Source: CAD feature listing. Evaluate the final solid. Frame: model axes, mm. Face numbers are marked on the shaded views. A direction names the side the tool comes from. Coordinates: 2 decimals unless noted, no trailing zeros. Loops run counter-clockwise (first coordinate to the right, second up) from the corner with the lowest first, then second, coordinate; pieces in that order, holes last. Notation, with made-up numbers: (50.5, 34.5) -> (94.5, 34.5) arc R22 cw to (94.5, 40.5) -> close; hole circle Ø3 at (-32.5, 82). An arc over 180 degrees is marked (long way). Answer as a JSON object with one key per item and string values. Group by question number.
from build123d import *

# Parameters (mm, degrees)
SKETCH_W        = 150
SKETCH_H        = 100
PAD_DEPTH       = 60
POCKET_DEPTH    = 58
SKETCH002_R     = 3
PAD001_DEPTH    = 37.8
POCKET001_DEPTH = 2
POCKET002_DEPTH = 2
SKETCH007_R     = 1
POCKET003_DEPTH = 2.001
SKETCH009_R     = 1.5
PAD003_DEPTH    = 10
POCKET004_DEPTH = 6
POCKET005_DEPTH = 6
CHAMFER_ANGLE   = 60
CHAMFER_SIZE    = 4
FILLET_R        = 2
FILLET001_R     = 2


with BuildPart() as part:
    # Sketch → Pad (new body)
    with BuildSketch(Plane.XZ):
        with Locations((75, 50)):
            Rectangle(SKETCH_W, SKETCH_H)
    extrude(amount=PAD_DEPTH)

    # Sketch001 (on Face6 of Pad) → Pocket (cut)
    with BuildSketch(Plane.XZ.offset(60)):
        Polygon((2, 98), (148, 98), (148, 56), (142, 56), (142, 44), (148, 44), (148, 2), (2, 2), (2, 44), (8, 44), (8, 56), (2, 56), align=None)
    extrude(amount=-POCKET_DEPTH, mode=Mode.SUBTRACT)

    # Sketch002 (on Face19 of Pocket) → Pad001 (join)
    with BuildSketch(Plane.XZ.offset(2)):
        with Locations((24.75, 80)):
            Circle(SKETCH002_R)
        with Locations((95.75, 80)):
            Circle(SKETCH002_R)
        with Locations((24.75, 20)):
            Circle(SKETCH002_R)
        with Locations((95.75, 20)):
            Circle(SKETCH002_R)
    extrude(amount=PAD001_DEPTH)

    # Sketch005 → Pocket001 (cut)
    with BuildSketch(Plane(origin=(0, 0, 0), x_dir=(1, 0, 0), z_dir=(0, 0, -1))):
        with BuildLine():
            ThreePointArc((65, 13), (61, 9), (65, 5))
            Line((65, 5), (85, 5))
            ThreePointArc((85, 5), (89, 9), (85, 13))
            Line((65, 13), (85, 13))
        make_face()
    extrude(amount=-POCKET001_DEPTH, mode=Mode.SUBTRACT)

    # Sketch006 (on Face5 of Pocket001) → Pocket002 (cut)
    with BuildSketch(Plane(origin=(150, 0, 0), x_dir=(0, 0, 1), z_dir=(1, 0, 0))):
        with BuildLine():
            ThreePointArc((25, 35), (17.5, 42.5), (10, 35))
            Line((10, 35), (10, 25))
            ThreePointArc((10, 25), (17.5, 17.5), (25, 25))
            Line((25, 35), (25, 25))
        make_face()
    extrude(amount=-POCKET002_DEPTH, mode=Mode.SUBTRACT)

    # Sketch007 (on Face27 of Pocket002) → Pocket003 (cut, through all)
    with BuildSketch(Plane.XZ.offset(2)):
        with Locations((40, 50)):
            Circle(SKETCH007_R)
        with Locations((110, 50)):
            Circle(SKETCH007_R)
    extrude(amount=-POCKET003_DEPTH, mode=Mode.SUBTRACT)

    # Sketch009 (on Face35 of Pocket003) → Pad003 (join)
    with BuildSketch(Plane.XZ.offset(39.8)):
        with Locations((24.75, 80)):
            Circle(SKETCH009_R)
        with Locations((95.75, 80)):
            Circle(SKETCH009_R)
        with Locations((24.75, 20)):
            Circle(SKETCH009_R)
        with Locations((95.75, 20)):
            Circle(SKETCH009_R)
    extrude(amount=PAD003_DEPTH)

    # Sketch010 (on Face14 of Pad003) → Pocket004 (cut)
    with BuildSketch(Plane(origin=(0, 0, 56), x_dir=(-1, 0, 0), z_dir=(0, 0, 1))):
        Polygon((-3.75, 60), (-3.75, 57.3), (-2.75, 57.3), (-2.75, 51.7), (-7.25, 51.7), (-7.25, 57.3), (-6.25, 57.3), (-6.25, 60), align=None)
    extrude(amount=-POCKET004_DEPTH, mode=Mode.SUBTRACT)

    # Sketch011 (on Face24 of Pocket004) → Pocket005 (cut)
    with BuildSketch(Plane(origin=(0, 0, 56), x_dir=(-1, 0, 0), z_dir=(0, 0, 1))):
        Polygon((-143.75, 60), (-146.25, 60), (-146.25, 57.3), (-147.25, 57.3), (-147.25, 51.7), (-142.74998, 51.7), (-142.75, 57.3), (-143.75, 57.3), align=None)
    extrude(amount=-POCKET005_DEPTH, mode=Mode.SUBTRACT)

    # Chamfer
    chamfer_edges = [part.edges().sort_by_distance(p)[0] for p in [
        (21.75, -2, 80),
        (92.75, -2, 80),
        (92.75, -2, 20),
        (21.75, -2, 20),
    ]]
    chamfer_side = part.faces().sort_by_distance((75.121299, -2, 50))[0]
    chamfer(chamfer_edges, length=CHAMFER_SIZE, angle=CHAMFER_ANGLE, reference=chamfer_side)

    # Fillet
    fillet_edges = [part.edges().sort_by_distance(p)[0] for p in [
        (2, -31, 98),
        (2, -31, 2),
        (148, -31, 2),
        (148, -31, 98),
    ]]
    fillet(fillet_edges, radius=FILLET_R)

    # Fillet001
    fillet001_edges = [part.edges().sort_by_distance(p)[0] for p in [
        (0, -30, 0),
        (0, -30, 100),
        (150, -30, 100),
        (150, -30, 0),
    ]]
    fillet(fillet001_edges, radius=FILLET001_R)


solid = part.part
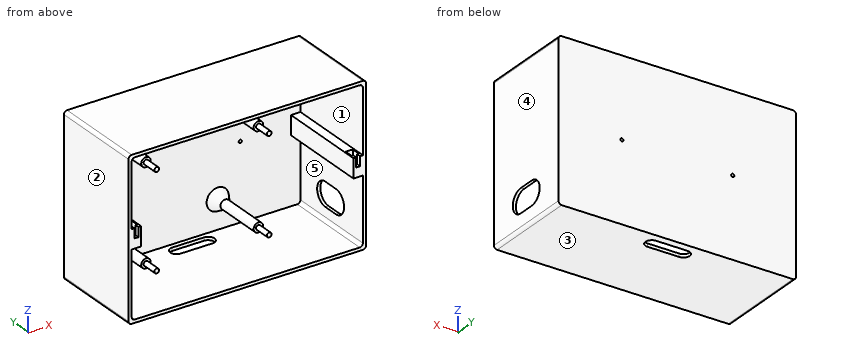
1. Reachability of the marked faces 1 and 2 from +Z, -Z, +X, -X, +Y, -Y: full face, straight path, thin tool, end or side. Return the list, or none.
2. Section query C-C on z = 35. Return loops of the section in (x, y).
3. Section query B-B on x = 80.5. Return loops of the section in (y, z).
4. Section query A-A on y = -48. Return loops of the section in (x, z).
5. Pin query (flat end, axial travel): pin 1 Ø1.8 at (x, z) = (110, 50) entering from -Y; pin 2 Ø3.5 at (x, z) = (25, 19.5) entering from -Y; pin 3 Ø4 at (x, z) = (53, 37.5) entering from -Y; pin 4 Ø1.3 at (x, z) = (5.5, 52.5) entering from -Y. Return the tip coordinate at first contact, or that it passes through.
6. Mould query, pull axis Z, two halves, no side actions, for the marked faces 3, 4 and 5. Classes: pulls with the +Z half, pulls with the -Z half, needs draft (parallel to the pull), parting line crosses it, or undercut.
7. Section query D-D on x = 12.5. Return loops of the section in (y, z), then the cut area to 3 significant figures.
8. Ray query, L1, parallel to Z at x = 18.5, y = -32.5; L2, parallel to X at y = -11.5, z = 50.5; L3, parallel to Z at x = 40, y = -0.5. Return the intervals inside material, ascending.
Solved:
{
 "1": {"face 1": "-Y", "face 2": "+Z, -Z, -X, +Y, -Y"},
 "2": {"outline": "(0, -60) -> (2, -60) -> (2, -2) -> (148, -2) -> (148, -60) -> (150, -60) -> (150, 0) -> (0, 0) -> close"},
 "3": {"outline": "(-60, 0) -> (-13, 0) -> (-13, 2) -> (-60, 2) -> close; (-60, 98) -> (-2, 98) -> (-2, 2) -> (-5, 2) -> (-5, 0) -> (0, 0) -> (0, 100) -> (-60, 100) -> close"},
 "4": {"outline": "(0, 2) arc R2 ccw to (2, 0) -> (148, 0) arc R2 ccw to (150, 2) -> (150, 98) arc R2 ccw to (148, 100) -> (2, 100) arc R2 ccw to (0, 98) -> close; circle Ø3 at (24.75, 20); circle Ø3 at (24.75, 80); circle Ø3 at (95.75, 20); circle Ø3 at (95.75, 80); hole (2, 4) arc R2 ccw to (4, 2) -> (146, 2) arc R2 ccw to (148, 4) -> (148, 44) -> (142, 44) -> (142, 56) -> (148, 56) -> (148, 96) arc R2 ccw to (146, 98) -> (4, 98) arc R2 ccw to (2, 96) -> (2, 56) -> (8, 56) -> (8, 44) -> (2, 44) -> close"},
 "5": {"pin 1": "through", "pin 2": "y = -49.8", "pin 3": "y = -2", "pin 4": "y = -51.7"},
 "6": {"face 3": "pulls with the -Z half", "face 4": "needs draft", "face 5": "undercut"},
 "7": {"outline": "(-60, 0) -> (0, 0) -> (0, 100) -> (-60, 100) -> (-60, 98) -> (-2, 98) -> (-2, 2) -> (-60, 2) -> close", "area": "432 mm^2"},
 "8": {"L1": "0 to 2, 98 to 100", "L2": "0 to 8, 142 to 150", "L3": "0 to 49, 51 to 100"}
}
